```python
from build123d import *

# Parameters (mm, degrees)
F0_W     = 267
F0_H     = 67.998115
F0_W_2   = 21
F0_H_2   = 21
F0_W_3   = 19
F0_H_3   = 19
F0_W_4   = 17
F0_H_4   = 17
F0_W_5   = 15
F0_H_5   = 15
F0_W_6   = 13
F0_H_6   = 13
F0_W_7   = 11
F0_H_7   = 11
F0_W_8   = 9
F0_H_8   = 9
F0_W_9   = 8
F0_H_9   = 8
F0_W_10  = 10
F0_H_10  = 10
F0_W_11  = 12
F0_H_11  = 12
F0_W_12  = 14
F0_H_12  = 14
F0_W_13  = 16
F0_H_13  = 16
F0_W_14  = 18
F0_H_14  = 18
F0_W_15  = 20
F0_H_15  = 20
F0_R     = 4.5
F0_R_2   = 5.5
F0_R_3   = 6.5
F0_R_4   = 7.5
F0_R_5   = 8.5
F0_R_6   = 9.5
F0_R_7   = 10.5
F0_R_8   = 10
F0_R_9   = 9
F0_R_10  = 8
F0_R_11  = 7
F0_R_12  = 6
F0_R_13  = 5
F0_R_14  = 4
F1_DEPTH = 1.5


with BuildPart() as f1:
    # F0 (on Front) → F1 (new body)
    with BuildSketch(Plane.XZ):
        with Locations((-5.5, 27.999057)):
            Rectangle(F0_W, F0_H)
        with Locations((-122.5, 10.5)):
            Rectangle(F0_W_2, F0_H_2, mode=Mode.SUBTRACT)
        with Locations((-98.5, 9.5)):
            Rectangle(F0_W_3, F0_H_3, mode=Mode.SUBTRACT)
        with Locations((-76.5, 8.5)):
            Rectangle(F0_W_4, F0_H_4, mode=Mode.SUBTRACT)
        with Locations((-56.5, 7.5)):
            Rectangle(F0_W_5, F0_H_5, mode=Mode.SUBTRACT)
        with Locations((-38.5, 6.5)):
            Rectangle(F0_W_6, F0_H_6, mode=Mode.SUBTRACT)
        with Locations((-22.5, 5.5)):
            Rectangle(F0_W_7, F0_H_7, mode=Mode.SUBTRACT)
        with Locations((-8.5, 4.5)):
            Rectangle(F0_W_8, F0_H_8, mode=Mode.SUBTRACT)
        with Locations((4, 4)):
            Rectangle(F0_W_9, F0_H_9, mode=Mode.SUBTRACT)
        with Locations((17, 5)):
            Rectangle(F0_W_10, F0_H_10, mode=Mode.SUBTRACT)
        with Locations((32, 6)):
            Rectangle(F0_W_11, F0_H_11, mode=Mode.SUBTRACT)
        with Locations((49, 7)):
            Rectangle(F0_W_12, F0_H_12, mode=Mode.SUBTRACT)
        with Locations((68, 8)):
            Rectangle(F0_W_13, F0_H_13, mode=Mode.SUBTRACT)
        with Locations((89, 9)):
            Rectangle(F0_W_14, F0_H_14, mode=Mode.SUBTRACT)
        with Locations((112, 10)):
            Rectangle(F0_W_15, F0_H_15, mode=Mode.SUBTRACT)
        with Locations((-128.5, 30.5)):
            Circle(F0_R, mode=Mode.SUBTRACT)
        with Locations((-114.5, 30.5)):
            Circle(F0_R_2, mode=Mode.SUBTRACT)
        with Locations((-98.5, 30.5)):
            Circle(F0_R_3, mode=Mode.SUBTRACT)
        with Locations((-80.5, 30.5)):
            Circle(F0_R_4, mode=Mode.SUBTRACT)
        with Locations((-60.5, 30.5)):
            Circle(F0_R_5, mode=Mode.SUBTRACT)
        with Locations((-38.5, 30.5)):
            Circle(F0_R_6, mode=Mode.SUBTRACT)
        with Locations((-14.5, 30.5)):
            Circle(F0_R_7, mode=Mode.SUBTRACT)
        Polygon((-122.5, 37.811581), (-133, 55.998115), (-112, 55.998115), align=None, mode=Mode.SUBTRACT)
        Polygon((-98.5, 39.543632), (-108, 55.998115), (-89, 55.998115), align=None, mode=Mode.SUBTRACT)
        Polygon((-76.5, 41.275683), (-85, 55.998115), (-68, 55.998115), align=None, mode=Mode.SUBTRACT)
        Polygon((-56.5, 43.007733), (-64, 55.998115), (-49, 55.998115), align=None, mode=Mode.SUBTRACT)
        Polygon((-38.5, 44.739784), (-45, 55.998115), (-32, 55.998115), align=None, mode=Mode.SUBTRACT)
        Polygon((-22.5, 46.471835), (-28, 55.998115), (-17, 55.998115), align=None, mode=Mode.SUBTRACT)
        Polygon((-8.5, 48.203886), (-13, 55.998115), (-4, 55.998115), align=None, mode=Mode.SUBTRACT)
        with Locations((10, 30.5)):
            Circle(F0_R_8, mode=Mode.SUBTRACT)
        with Locations((33, 30.5)):
            Circle(F0_R_9, mode=Mode.SUBTRACT)
        with Locations((54, 30.5)):
            Circle(F0_R_10, mode=Mode.SUBTRACT)
        with Locations((73, 30.5)):
            Circle(F0_R_11, mode=Mode.SUBTRACT)
        with Locations((90, 30.5)):
            Circle(F0_R_12, mode=Mode.SUBTRACT)
        with Locations((105, 30.5)):
            Circle(F0_R_13, mode=Mode.SUBTRACT)
        with Locations((118, 30.5)):
            Circle(F0_R_14, mode=Mode.SUBTRACT)
        Polygon((4, 49.069911), (0, 55.998115), (8, 55.998115), align=None, mode=Mode.SUBTRACT)
        Polygon((17, 47.33786), (12, 55.998115), (22, 55.998115), align=None, mode=Mode.SUBTRACT)
        Polygon((32, 45.60581), (26, 55.998115), (38, 55.998115), align=None, mode=Mode.SUBTRACT)
        Polygon((49, 43.873759), (42, 55.998115), (56, 55.998115), align=None, mode=Mode.SUBTRACT)
        Polygon((68, 42.141708), (60, 55.998115), (76, 55.998115), align=None, mode=Mode.SUBTRACT)
        Polygon((89, 40.409657), (80, 55.998115), (98, 55.998115), align=None, mode=Mode.SUBTRACT)
        Polygon((112, 38.677606), (102, 55.998115), (122, 55.998115), align=None, mode=Mode.SUBTRACT)
    extrude(amount=F1_DEPTH)


solid = f1.part
```
Here's how the part is built. I have some questions about the finished solid (model axes, mm). Coordinates: 2 decimals unless noted, no trailing zeros. Order: outer loops, then holes, each group sorted by start corner. A loop starts at its lowest first (then second) coordinate and runs counter-clockwise, first axis right, second up. Notation, with made-up numbers: (-35.75, -36) -> (3.25, -36) arc R13 cw to (3.25, -30) -> close; hole circle Ø7 at (4.5, 43.5). An arc over 180 degrees is marked (long way). Return JSON: item names as keys, results as strings.
1) If we section it at D-D on x = 118: List the corners of the cut face in (y, z) for me, plus the area to 3 significant figures.
Conclusion:
{"outline": "(-1.5, -6) -> (0, -6) -> (0, 0) -> (-1.5, 0) -> close; (-1.5, 20) -> (0, 20) -> (0, 26.5) -> (-1.5, 26.5) -> close; (-1.5, 34.5) -> (0, 34.5) -> (0, 49.07) -> (-1.5, 49.07) -> close; (-1.5, 56) -> (0, 56) -> (0, 62) -> (-1.5, 62) -> close", "area": "49.6 mm²"}
2) If I drill on probe 1 along Z at (x, y) = (-81, -1.15); probe 2 along Z at (x, y) = (-114.5, -1); probe 3 along Z at (x, y) = (10, -0.6), over which ranges is the centre line in solid material (lowest first)?
Conclusion:
{"probe 1": "z = -6 to 0, 17 to 23.02, 37.98 to 49.07, 56 to 62", "probe 2": "z = -6 to 0, 21 to 25, 36 to 51.67, 56 to 62", "probe 3": "z = -6 to 20.5, 40.5 to 62"}
3) I'm going to push a flat-ended pin straight in: P1, Ø3, axis at x = -56.5, z = 49, coming from the +Y side. Where does the tip first touch, or does it pass through?
Conclusion:
{"P1": "passes through"}
4) If we section it at A-A on x = -128.5: List the corners of the cut face in (y, z) for me, plus the area to 3 significant figures.
Conclusion:
{"outline": "(-1.5, -6) -> (0, -6) -> (0, 0) -> (-1.5, 0) -> close; (-1.5, 21) -> (0, 21) -> (0, 26) -> (-1.5, 26) -> close; (-1.5, 35) -> (0, 35) -> (0, 48.2) -> (-1.5, 48.2) -> close; (-1.5, 56) -> (0, 56) -> (0, 62) -> (-1.5, 62) -> close", "area": "45.3 mm²"}
5) Thinking about a two-plate mould opening in X: for faces 1 (the cylindrical face through (-92.3, -0.74, 32.45)), 2 (the cylindrical face through (7.83, -0.74, 20.74)), which applies, +X half, -X half, draft (parallel to the pull), parting line (faces both ways), or undercut?
Conclusion:
{"face 1": "undercut", "face 2": "undercut"}
6) If we section it at B-B on y = -1.2: State how many separate pieces and enclosed holes the cut face has, plus the area to 3 significant figures.
Conclusion:
{"separate pieces": "1", "enclosed holes": "42", "area": "11,100 mm²"}
